from build123d import *
from OCP.BRepFilletAPI import BRepFilletAPI_MakeFillet

# Parameters (mm, degrees)
SKETCH1_W              = 41.97
SKETCH1_H              = 32.5
BOSS_EXTRUDE1_DEPTH    = 0.75
SKETCH2_W              = 41.97
SKETCH2_H              = 21.7
BOSS_EXTRUDE2_DEPTH    = 1.75
SKETCH4_W              = 2.75
SKETCH4_H              = 21.7
BOSS_EXTRUDE3_DEPTH    = 31.5
SKETCH5_W              = 21.7
SKETCH5_H              = 12
CUT_EXTRUDE1_DEPTH     = 1.6
SKETCH6_W              = 32.5
SKETCH6_H              = 9.2
BOSS_EXTRUDE4_DEPTH    = 1.15
SKETCH7_W              = 41.97
SKETCH7_H              = 21.7
BOSS_EXTRUDE5_DEPTH    = 1
SKETCH8_W              = 41.97
SKETCH8_H              = 40
BOSS_EXTRUDE6_DEPTH    = 1
FILLET1_R              = 4
FILLET1_R_2            = 2
FILLET1_R_3            = 1
FILLET1_OF_MIRROR2_R   = 4
FILLET1_OF_MIRROR2_R_2 = 2
FILLET1_OF_MIRROR2_R_3 = 1
FILLET2_R              = 1
SKETCH9_W              = 41.97
SKETCH9_H              = 1.5
BOSS_EXTRUDE7_DEPTH    = 4
FILLET4_R              = 4
FILLET5_R              = 2


with BuildPart() as part:
    # Sketch1 → Boss-Extrude1 (new, symmetric)
    with BuildSketch(Plane(origin=(0, 0, 0), x_dir=(1, 0, 0), z_dir=(0, 1, 0))):
        Rectangle(SKETCH1_W, SKETCH1_H)
    extrude(amount=BOSS_EXTRUDE1_DEPTH, both=True)

    # Sketch2 → Boss-Extrude2 (add, symmetric)
    with BuildSketch(Plane(origin=(0, 0, 0), x_dir=(1, 0, 0), z_dir=(0, 1, 0))):
        Rectangle(SKETCH2_W, SKETCH2_H)
    extrude(amount=BOSS_EXTRUDE2_DEPTH, both=True)

    # Sketch4 → Boss-Extrude3 (add)
    with BuildSketch(Plane(origin=(0, 0.75, 0), x_dir=(1, 0, 0), z_dir=(0, 1, 0))):
        with Locations((-19.61, 0)):
            Rectangle(SKETCH4_W, SKETCH4_H)
    boss_extrude3 = extrude(amount=BOSS_EXTRUDE3_DEPTH)

    # Sketch5 → Cut-Extrude1 (cut)
    with BuildSketch(Plane(origin=(-18.235, 0, 0), x_dir=(0, 0, -1), z_dir=(1, 0, 0))):
        with Locations((0, 17)):
            Rectangle(SKETCH5_W, SKETCH5_H)
    cut_extrude1 = extrude(amount=-CUT_EXTRUDE1_DEPTH, mode=Mode.SUBTRACT)

    # Sketch6 → Boss-Extrude4 (add)
    with BuildSketch(Plane(origin=(-19.835, 0, 0), x_dir=(0, 0, -1), z_dir=(1, 0, 0))):
        with Locations((0, 17)):
            Rectangle(SKETCH6_W, SKETCH6_H)
    boss_extrude4 = extrude(amount=-BOSS_EXTRUDE4_DEPTH)

    # Sketch7 → Boss-Extrude5 (add)
    with BuildSketch(Plane(origin=(0, 32.25, 0), x_dir=(1, 0, 0), z_dir=(0, 1, 0))):
        Rectangle(SKETCH7_W, SKETCH7_H)
    boss_extrude5 = extrude(amount=BOSS_EXTRUDE5_DEPTH)

    # Sketch8 → Boss-Extrude6 (add)
    with BuildSketch(Plane(origin=(0, 33.25, 0), x_dir=(1, 0, 0), z_dir=(0, 1, 0))):
        with Locations((0, 0.25)):
            Rectangle(SKETCH8_W, SKETCH8_H)
    boss_extrude6 = extrude(amount=BOSS_EXTRUDE6_DEPTH)

    # Fillet1
    fillet1_edges_1 = [part.edges().sort_by_distance(p)[0] for p in [
        (20.985, 33.75, -20.25),
    ]]
    fillet1_edges_2 = [part.edges().sort_by_distance(p)[0] for p in [
        (-20.985, 33.75, -20.25),
        (-20.985, 33.75, 19.75),
        (20.985, 33.75, 19.75),
    ]]
    fillet1_edges_3 = [part.edges().sort_by_distance(p)[0] for p in [
        (20.985, 32.25, 0),
        (1.375, 32.25, 10.85),
        (1.375, 32.25, -10.85),
    ]]
    fillet1 = BRepFilletAPI_MakeFillet(part.part.solid().wrapped)
    for e in fillet1_edges_1:
        fillet1.Add(FILLET1_R - 0.0001, e.wrapped)
    for e in fillet1_edges_2:
        fillet1.Add(FILLET1_R_2 - 0.0001, e.wrapped)
    for e in fillet1_edges_3:
        fillet1.Add(FILLET1_R_3 - 0.0001, e.wrapped)
    add(Compound.cast(fillet1.Shape()), mode=Mode.REPLACE)  # a hair under: the kernel refuses the full size

    # Mirror2: Boss-Extrude3, Cut-Extrude1, Boss-Extrude4, Boss-Extrude5, Boss-Extrude6 across plane
    add(boss_extrude3.mirror(Plane.ZX))
    add(cut_extrude1.mirror(Plane.ZX), mode=Mode.SUBTRACT)
    add(boss_extrude4.mirror(Plane.ZX))
    add(boss_extrude5.mirror(Plane.ZX))
    add(boss_extrude6.mirror(Plane.ZX))

    # Fillet1 of Mirror2
    fillet1_of_mirror2_edges_1 = [part.edges().sort_by_distance(p)[0] for p in [
        (20.985, -33.75, -20.25),
    ]]
    fillet1_of_mirror2_edges_2 = [part.edges().sort_by_distance(p)[0] for p in [
        (-20.985, -33.75, -20.25),
        (-20.985, -33.75, 19.75),
        (20.985, -33.75, 19.75),
    ]]
    fillet1_of_mirror2_edges_3 = [part.edges().sort_by_distance(p)[0] for p in [
        (20.985, -32.25, 0),
        (1.375, -32.25, 10.85),
        (1.375, -32.25, -10.85),
    ]]
    fillet1_of_mirror2 = BRepFilletAPI_MakeFillet(part.part.solid().wrapped)
    for e in fillet1_of_mirror2_edges_1:
        fillet1_of_mirror2.Add(FILLET1_OF_MIRROR2_R - 0.0001, e.wrapped)
    for e in fillet1_of_mirror2_edges_2:
        fillet1_of_mirror2.Add(FILLET1_OF_MIRROR2_R_2 - 0.0001, e.wrapped)
    for e in fillet1_of_mirror2_edges_3:
        fillet1_of_mirror2.Add(FILLET1_OF_MIRROR2_R_3 - 0.0001, e.wrapped)
    add(Compound.cast(fillet1_of_mirror2.Shape()), mode=Mode.REPLACE)  # a hair under: the kernel refuses the full size

    # Fillet2
    fillet2_edges = [part.edges().sort_by_distance(p)[0] for p in [
        (20.985, -1.75, 0),
        (20.985, 1.75, 0),
        (1.375, -1.75, 10.85),
        (1.375, -1.75, -10.85),
        (1.375, 1.75, 10.85),
        (1.375, 1.75, -10.85),
    ]]
    fillet(fillet2_edges, radius=FILLET2_R - 0.0001)  # a hair under: the kernel refuses the full size

    # Sketch9 → Boss-Extrude7 (add)
    with BuildSketch(Plane(origin=(0, 0, -16.25), x_dir=(-1, 0, 0), z_dir=(0, 0, -1))):
        Rectangle(SKETCH9_W, SKETCH9_H)
    extrude(amount=BOSS_EXTRUDE7_DEPTH)

    # Fillet4
    fillet4_edges = [part.edges().sort_by_distance(p)[0] for p in [
        (20.985, 0, -20.25),
    ]]
    fillet(fillet4_edges, radius=FILLET4_R)

    # Fillet5
    fillet5_edges = [part.edges().sort_by_distance(p)[0] for p in [
        (-20.985, 0, -20.25),
    ]]
    fillet(fillet5_edges, radius=FILLET5_R)


solid = part.part
Work out the finished part from the listing and answer in its coordinate system (mm). A direction names the side the tool comes from. Coordinates: 2 decimals unless noted, no trailing zeros. Loops run counter-clockwise (first coordinate to the right, second up) from the corner with the lowest first, then second, coordinate; pieces in that order, holes last. Notation, with made-up numbers: M -7.5,82 L 1.5,82 A24 ccw 1.5,119 Z; hole C 85,-40 d10. An arc over 180 degrees is marked long. Answer in a Markdown table with one row per item. Add a question column.
1. Find section D-D, the plane y = 15. Write down the section's boundary in (x, z) (3 decimals).
2. The mould has two halves that part along Y. Classify faces 1 (the cylindrical face through (-20.384, 0.01, -19.68)), 2 (the flat face through (0, -34.25, -1)), 3 (the flat face through (-20, 6, 10.85)): pulls with the +Y half, pulls with the -Y half, needs draft (parallel to the pull), parting line crosses it, or undercut.
3. A tool of negligible diameter and unlimited length cuts with its end or side. For faces 4 (the flat face through (0, 33.25, 15)), 5 (the flat face through (-19, -11, 0)), 6 (the flat face through (0, 0.75, -15)), from which of +Z, -Z, +X, -X, +Y, -Y can it reach the whole face along a straight path? Write none if from no direction.
4. Find section B-B, the plane x = 13. State how many separate pieces and enclosed holes the cut face has, then the cut area to 3 significant figures.
5. Find section C-C, the plane z = -0.5. Write down the section's boundary in (x, y) (3 decimals), then the cut area to 3 significant figures.
6. Flat-ended cylindrical pins translate along their axes: P1, Ø13, axis at x = 9, y = -6.5, coming from the +Z side; P2, Ø4, axis at y = -27, z = -3.5, coming from the +X side (3 decimals); P3, Ø13, axis at x = 2.5, y = 26, coming from the -Z side. Find the tip coordinate at first contact, or state that the pin passes through.
7. Consider L1, parallel to Y at x = 7.5, z = 10; L2, parallel to Y at x = -0.5, z = 1.5; L3, parallel to Y at x = -15, z = 18. Determine where each line is inside the solid, lowest interval first.
8. Find section A-A, the plane z = -12.5. Write down the section's boundary in (x, y) (3 decimals), then the cut area to 3 significant figures.
Reported:
| question | item | result |
|---|---|---|
| 1 | outline | M -20.985,-16.25 L -19.835,-16.25 L -19.835,16.25 L -20.985,16.25 Z |
| 2 | face 1 | needs draft |
| 2 | face 2 | pulls with the -Y half |
| 2 | face 3 | undercut |
| 3 | face 4 | +Z, +X, -X |
| 3 | face 5 | +Z, -Z, +X |
| 3 | face 6 | -Z, +X, -X |
| 4 | separate pieces | 3 |
| 4 | enclosed holes | 0 |
| 4 | area | 220 mm^2 |
| 5 | outline | M -20.985,-34.25 L 20.985,-34.25 L 20.985,-33.25 A1 ccw 19.985,-32.25 L -18.235,-32.25 L -18.235,-23 L -19.835,-23 L -19.835,-11 L -18.235,-11 L -18.235,-1.75 L 19.985,-1.75 A1 ccw 20.985,-0.75 L 20.985,0.75 A1 ccw 19.985,1.75 L -18.235,1.75 L -18.235,11 L -19.835,11 L -19.835,23 L -18.235,23 L -18.235,32.25 L 19.985,32.25 A1 ccw 20.985,33.25 L 20.985,34.25 L -20.985,34.25 Z |
| 5 | area | 443 mm^2 |
| 6 | P1 | stops at z = 16.25 |
| 6 | P2 | stops at x = -18.235 |
| 6 | P3 | stops at z = -10.51 |
| 7 | L1 | y = -34.25 to -32.26, -1.74 to 1.74, 32.26 to 34.25 |
| 7 | L2 | y = -34.25 to -32.25, -1.75 to 1.75, 32.25 to 34.25 |
| 7 | L3 | y = -34.25 to -33.25, 33.25 to 34.25 |
| 8 | outline | M -20.985,-34.25 L 20.985,-34.25 L 20.985,-33.25 L -20.985,-33.25 Z; M -20.985,-21.6 L -19.835,-21.6 L -19.835,-12.4 L -20.985,-12.4 Z; M -20.985,-0.75 L 20.985,-0.75 L 20.985,0.75 L -20.985,0.75 Z; M -20.985,12.4 L -19.835,12.4 L -19.835,21.6 L -20.985,21.6 Z; M -20.985,33.25 L 20.985,33.25 L 20.985,34.25 L -20.985,34.25 Z |
| 8 | area | 168 mm^2 |
